```python
from build123d import *

# Parameters (mm, degrees)
BOSS_EXTRUDE1_DEPTH = 6


with BuildPart() as part:
    # Model → Boss-Extrude1 (new body)
    with BuildSketch(Plane.XY):
        Polygon((0, 203), (0, 181), (6, 181), (6, 169), (0, 169), (0, 157), (6, 157), (6, 145), (0, 145), (0, 133), (6, 133), (6, 121), (0, 121), (0, 109), (6, 109), (6, 97), (0, 97), (0, 85), (6, 85), (6, 73), (0, 73), (0, 61), (6, 61), (6, 49), (0, 49), (0, 37), (6, 37), (6, 25), (0, 25), (0, 13), (0, 3), (22, 3), (22, 9), (34, 9), (34, 3), (46, 3), (46, 9), (58, 9), (58, 3), (70, 3), (70, 9), (82, 9), (82, 3), (94, 3), (94, 9), (106, 9), (106, 3), (118, 3), (118, 9), (130, 9), (130, 3), (142, 3), (142, 9), (154, 9), (154, 3), (166, 3), (166, 9), (178, 9), (178, 3), (190, 3), (200, 3), (200, 25), (194, 25), (194, 37), (200, 37), (200, 49), (194, 49), (194, 61), (200, 61), (200, 73), (194, 73), (194, 85), (200, 85), (200, 97), (194, 97), (194, 109), (200, 109), (200, 121), (194, 121), (194, 133), (200, 133), (200, 145), (194, 145), (194, 157), (200, 157), (200, 169), (194, 169), (194, 181), (200, 181), (200, 193), (200, 203), (178, 203), (178, 197), (166, 197), (166, 203), (154, 203), (154, 197), (142, 197), (142, 203), (130, 203), (130, 197), (118, 197), (118, 203), (106, 203), (106, 197), (94, 197), (94, 203), (82, 203), (82, 197), (70, 197), (70, 203), (58, 203), (58, 197), (46, 197), (46, 203), (34, 203), (34, 197), (22, 197), (22, 203), (10, 203), align=None)
    extrude(amount=BOSS_EXTRUDE1_DEPTH)


solid = part.part
```
Can you work these out from the model? Positions are in its coordinate system, mm. A direction names the side the tool comes from. Give positions to 0.01 mm unless a question says otherwise; leave off trailing zeros. Loops run counter-clockwise (first coordinate to the right, second up) from the corner with the lowest first, then second, coordinate; pieces in that order, holes last. Notation, with made-up numbers: M 55,33 L 103,33 A19 ccw 103,46 Z; hole C -3,20 d3. An arc over 180 degrees is marked long. Use CSV: the item, a comma, the result in double quotes. Start each with the question number.
1. On a 3-axis mill with a long thin cutter (end or side, diameter ignored), from which of +Z, -Z, +X, -X, +Y, -Y can I reach the whole of each face in a straight line? I mean faces 4 (the face through (28, 197, 3)), 5 (the face through (46, 6, 3)), 6 (the face through (197, 181, 3)). Say none if no direction works.
2. If I drill on L1, parallel to Y at x = 47, z = 4.1; L2, parallel to X at y = 128, z = 2.05, over which ranges is the centre line in solid material (lowest first)?
3. For P1, Ø3, axis at y = 198.5, z = 2.5, coming from the -X side; P2, Ø1, axis at y = 74, z = 4.5, coming from the +X side, each with a flat end and sliding along its axis, tell me the tip position at first contact or that it passes through.
4. Imagine slicing it at A-A, the plane y = 154. Write out the boundary of the cut face in (x, z).
5. Imagine slicing it at B-B, the plane x = 126. Write out the boundary of the cut face in (y, z).
6. If we mould it in two halves opening along Y, with no side actions, what happens to faces 1 (the face through (64, 203, 3)), 2 (the face through (197, 109, 3)), 3 (the face through (40, 3, 3))? For each: released by +Y, released by -Y, zero draft, split by the parting line, or undercut.
Response values:
1,face 4,"+Z, -Z, +Y"
1,face 5,"+Z, -Z, -Y"
1,face 6,"+Z, -Z, +X"
2,L1,"9 to 197"
2,L2,"6 to 194"
3,P1,"x = 0"
3,P2,"x = 194"
4,outline,"M 6,0 L 194,0 L 194,6 L 6,6 Z"
5,outline,"M 9,0 L 197,0 L 197,6 L 9,6 Z"
6,face 1,"released by +Y"
6,face 2,"undercut"
6,face 3,"released by -Y"
